Drawing for the job (mm, zero at the part's lowest x, y, z). A direction names the side the tool comes from. Give positions to 0.01 mm unless a question says otherwise; leave off trailing zeros. Loops run counter-clockwise (first coordinate to the right, second up) from the corner with the lowest first, then second, coordinate; pieces in that order, holes last. Notation, with made-up numbers: (-28, 37) -> (30, 37) arc R17 cw to (30, 42) -> close; hole circle Ø4 at (-32, 1.5). An arc over 180 degrees is marked (long way). Write item = value, one per line.
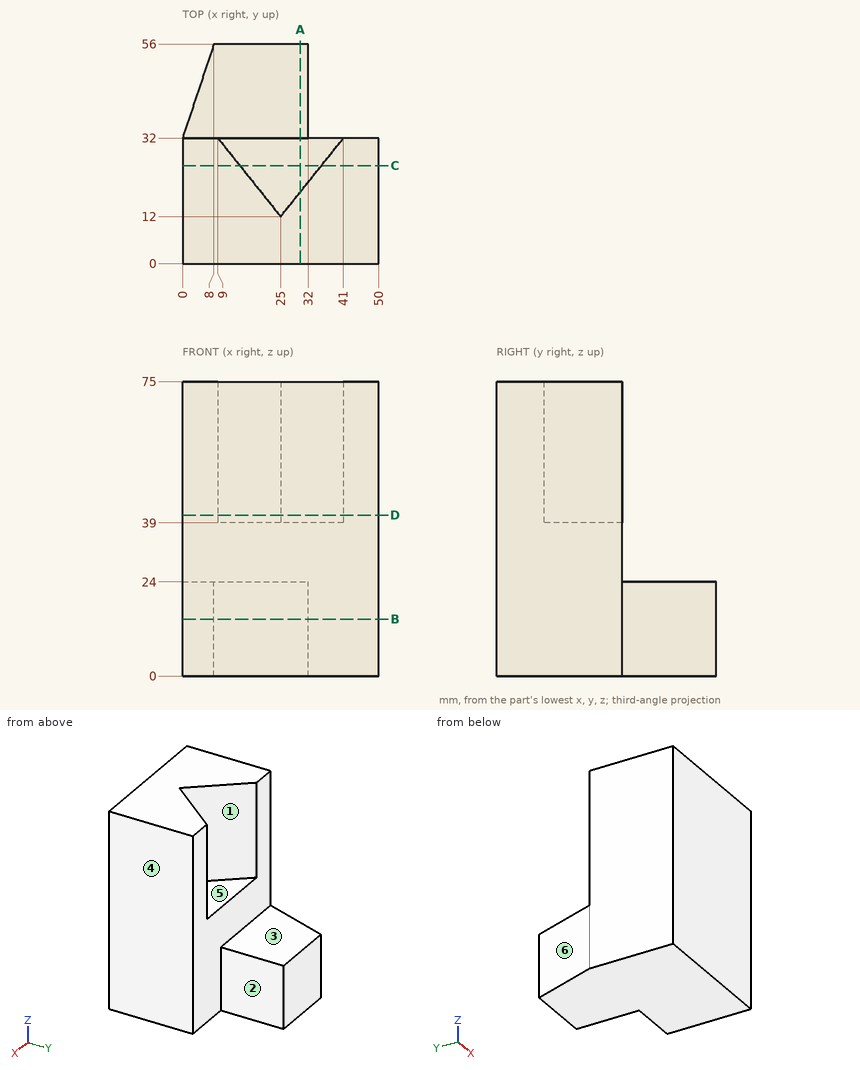
1) Slice it at B-B, the plane z = 14.5. List the corners of the cut face in (x, y), and give its area (3 significant figures).
Resolved:
outline = (0, 0) -> (50, 0) -> (50, 32) -> (32, 32) -> (32, 56) -> (8, 56) -> (0, 32) -> close
area = 2,270 mm²
2) Drill centre lines: line 1 along Y through (x, z) = (36, 33); line 2 along Z through (x, y) = (4, 38.5); line 3 along Z through (x, y) = (11, 31.5). Where is each one in solid material? Low to high. Write a range as [from, to].
Resolved:
line_1 = [0, 32]
line_2 = [0, 24]
line_3 = [0, 39]
3) Drop flat-ended pins along their axis: P1, Ø8, axis at x = 5.5, z = 35.5, coming from the +Y side; P2, Ø7, axis at y = 45, z = 10, coming from the +X side; P3, Ø6, axis at y = 47.5, z = 11, coming from the -X side. Give the stop position or say it passes through.
Resolved:
P1 = 32
P2 = 32
P3 = 4.17
4) Slice it at D-D, the plane z = 41. List the corners of the cut face in (x, y), and give its area (3 significant figures).
Resolved:
outline = (0, 0) -> (50, 0) -> (50, 32) -> (41, 32) -> (25, 12) -> (9, 32) -> (0, 32) -> close
area = 1,280 mm²
5) Slice it at A-A, the plane x = 30. List the corners of the cut face in (y, z), and give its area (3 significant figures).
Resolved:
outline = (0, 0) -> (56, 0) -> (56, 24) -> (32, 24) -> (32, 39) -> (18.25, 39) -> (18.25, 75) -> (0, 75) -> close
area = 2,480 mm²
6) Which spindle directions (+Z, -Z, +X, -X, +Y, -Y) get a long thin tool onto all of the face, cutting with end or side? Do the marked faces 1, 2 and 3. Say none if no direction does.
Resolved:
face_1 = +Z, +Y
face_2 = +Z, -Z, +X, +Y
face_3 = +Z, +X, -X, +Y
7) Pull direction X, two halves, no side cores. Call the marked faces 4, 5 and 6: pulls with the +X half, pulls with the -X half, needs draft (parallel to the pull), parting line crosses it, or undercut.
Resolved:
face_4 = pulls with the +X half
face_5 = undercut
face_6 = pulls with the -X half
8) Slice it at C-C, the plane y = 25. List the corners of the cut face in (x, z), and give its area (3 significant figures).
Resolved:
outline = (0, 0) -> (50, 0) -> (50, 75) -> (35.4, 75) -> (35.4, 39) -> (14.6, 39) -> (14.6, 75) -> (0, 75) -> close
area = 3,000 mm²
